Read the model definition and answer for the solid it produces. Units are mm, in the model's axes. Face numbers are marked on the shaded views. Round coordinates to 2 decimals unless told otherwise and drop trailing zeros. Order: outer loops, then holes, each group sorted by start corner. A loop starts at its lowest first (then second) coordinate and runs counter-clockwise, first axis right, second up. Notation, with made-up numbers: (54, 57.5) - (81, 57.5) arc R24 cw to (81, 77.5) - close; hole circle Ø1 at (-5.75, 28.5). An arc over 180 degrees is marked (long way). One line per question, with ' | ' between items. Start each with the question number.
1) The part is cut by section D-D, the plane x = -41. Give the vertices of the cut face in (y, z).
2) The mould has two halves that part along Z. Classify the marked faces 1, 2 and 3: pulls with the +Z half, pulls with the -Z half, needs draft (parallel to the pull), parting line crosses it, or undercut.
3) The part is cut by section C-C, the plane z = -107.5. Give the vertices of the cut face in (x, y), plus the area to 3 significant figures.
4) The part is cut by section A-A, the plane x = 0. Give the vertices of the cut face in (y, z).
5) Flat-ended cylindrical pins translate along their axes: pin 1 (4 mm diameter, centred on y = 23.5, z = -73, fed in from -X); pin 2 (4 mm diameter, centred on x = -30, y = 20.5, fed in from -Z); pin 3 (5 mm diameter, centred on y = 14.5, z = 85.5, fed in from +X); pin 4 (16 mm diameter, centred on x = 0, z = 0, fed in from +Y). Find the tip coordinate at first contact, or state that the pin passes through.
6) Straight lines are drawn through the part: line 1 (Z direction, x = 0, y = 20); line 2 (X direction, y = 22.25, z = 59); line 3 (Z direction, x = 0, y = 18.25). For each, find the intervals that lie inside material, in ascending order. Write a range as from..to.
7) The part is cut by section B-B, the plane z = 119. Give the vertices of the cut face in (x, y).
from build123d import *

# Parameters (mm, degrees)
SKETCH1_R           = 200
SKETCH1_R_2         = 180
EXTRUDE_THIN1_DEPTH = 30
SKETCH2_R           = 29.35
SKETCH2_R_2         = 9.35
EXTRUDE_THIN2_DEPTH = 10
BOSS_EXTRUDE1_DEPTH = 10
CIRPATTERN1_COUNT   = 5
SCALE3_SCALE        = 0.75


with BuildPart() as part:
    # Sketch1 → Extrude-Thin1 (new body)
    with BuildSketch(Plane(origin=(0, 0, 0), x_dir=(1, 0, 0), z_dir=(0, 1, 0))):
        Circle(SKETCH1_R)
        Circle(SKETCH1_R_2, mode=Mode.SUBTRACT)
    extrude(amount=EXTRUDE_THIN1_DEPTH)



with BuildPart() as body_2:
    # Sketch2 → Extrude-Thin2 (new body)
    with BuildSketch(Plane(origin=(0, 30, 0), x_dir=(1, 0, 0), z_dir=(0, 1, 0))):
        Circle(SKETCH2_R)
        Circle(SKETCH2_R_2, mode=Mode.SUBTRACT)
    extrude(amount=-EXTRUDE_THIN2_DEPTH)


with BuildPart() as part_1:
    add(part.part)

    add(body_2.part)  # Boss-Extrude1 merges body 2
    # Sketch3 → Boss-Extrude1 (add)
    with BuildSketch(Plane(origin=(0, 30, 0), x_dir=(1, 0, 0), z_dir=(0, 1, 0))):
        with BuildLine():
            Line((10, 29.35), (10, 180))
            ThreePointArc((10, 180), (0, 190), (-10, 180))
            Line((-10, 180), (-10, 29.35))
            ThreePointArc((-10, 29.35), (0, 19.35), (10, 29.35))
        make_face()
    boss_extrude1 = extrude(amount=-BOSS_EXTRUDE1_DEPTH)

    # CirPattern1: Boss-Extrude1 ×5 about axis
    cirpattern1_axis = Axis((0, 0, 0), (0, 1, 0))
    for i in range(1, CIRPATTERN1_COUNT):
        add(boss_extrude1.rotate(cirpattern1_axis, i * 360 / CIRPATTERN1_COUNT))


with BuildPart() as part_2:
    # Scale3: scaled about (0, 16.967452181, 0)
    add(part_1.part.scale(SCALE3_SCALE).moved(Location((0, 4.241863045, 0))))


solid = part_2.part
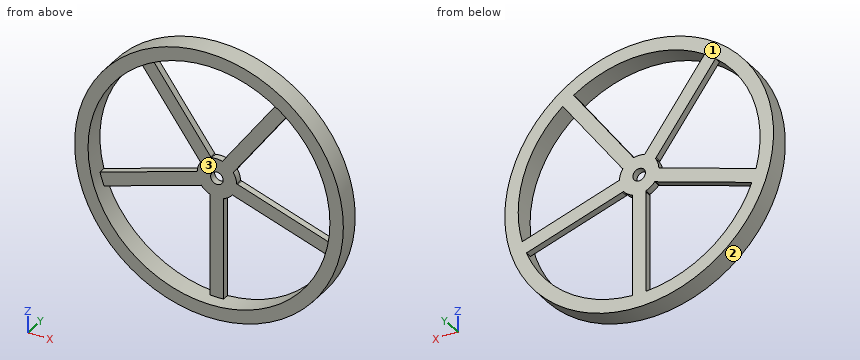
Values:
1) outline: (4.24, -144.29) - (26.74, -144.29) - (26.74, -128.62) - (4.24, -128.62) - close; (4.24, 128.62) - (26.74, 128.62) - (26.74, 144.29) - (4.24, 144.29) - close; (19.24, -21.21) - (26.74, -21.21) - (26.74, -5.44) - (19.24, -5.44) - close; (19.24, 43.67) - (26.74, 43.67) - (26.74, 69.19) - (19.24, 69.19) - close
2) face 1: needs draft | face 2: parting line crosses it | face 3: undercut
3) outline: (-104.61, 4.24) - (-81.66, 4.24) - (-81.66, 26.74) - (-104.61, 26.74) - close; (-7.5, 19.24) - (7.5, 19.24) - (7.5, 26.74) - (-7.5, 26.74) - close; (81.66, 4.24) - (104.61, 4.24) - (104.61, 26.74) - (81.66, 26.74) - close | area: 1,150 mm^2
4) outline: (4.24, -150) - (26.74, -150) - (26.74, -7.01) - (19.24, -7.01) - (19.24, -135) - (4.24, -135) - close; (4.24, 135) - (26.74, 135) - (26.74, 150) - (4.24, 150) - close; (19.24, 7.01) - (26.74, 7.01) - (26.74, 22.01) - (19.24, 22.01) - close
5) pin 1: stops at x = -132.13 | pin 2: stops at z = -147.36 | pin 3: stops at x = 124.94 | pin 4: stops at y = 26.74
6) line 1: z = -150..-7.01, 7.01..22.01, 135..150 | line 2: x = -137.91..-121.42, -52.14..-33.6, 33.6..52.14, 121.42..137.91 | line 3: z = -150..-135, 135..150
7) outline: (-91.32, 4.24) - (-63.75, 4.24) - (-63.75, 26.74) - (-91.32, 26.74) - close; (63.75, 4.24) - (91.32, 4.24) - (91.32, 26.74) - (63.75, 26.74) - close
